Print and shaded views of the part. All mm, measured from the part's lowest x, y and z. A direction names the side the tool comes from. Coordinates: 2 decimals unless noted, no trailing zeros. Write each loop counter-clockwise with the first axis right and the second up, starting at its lowest first coordinate (ties: lowest second). Pieces come first, ordered by that corner, then holes. Notation, with made-up numbers: (-28.5, 38.5) -> (20.5, 38.5) arc R21 cw to (20.5, 61.5) -> close; hole circle Ø9 at (78, -27). An arc over 180 degrees is marked (long way). Write item = value, one per line.
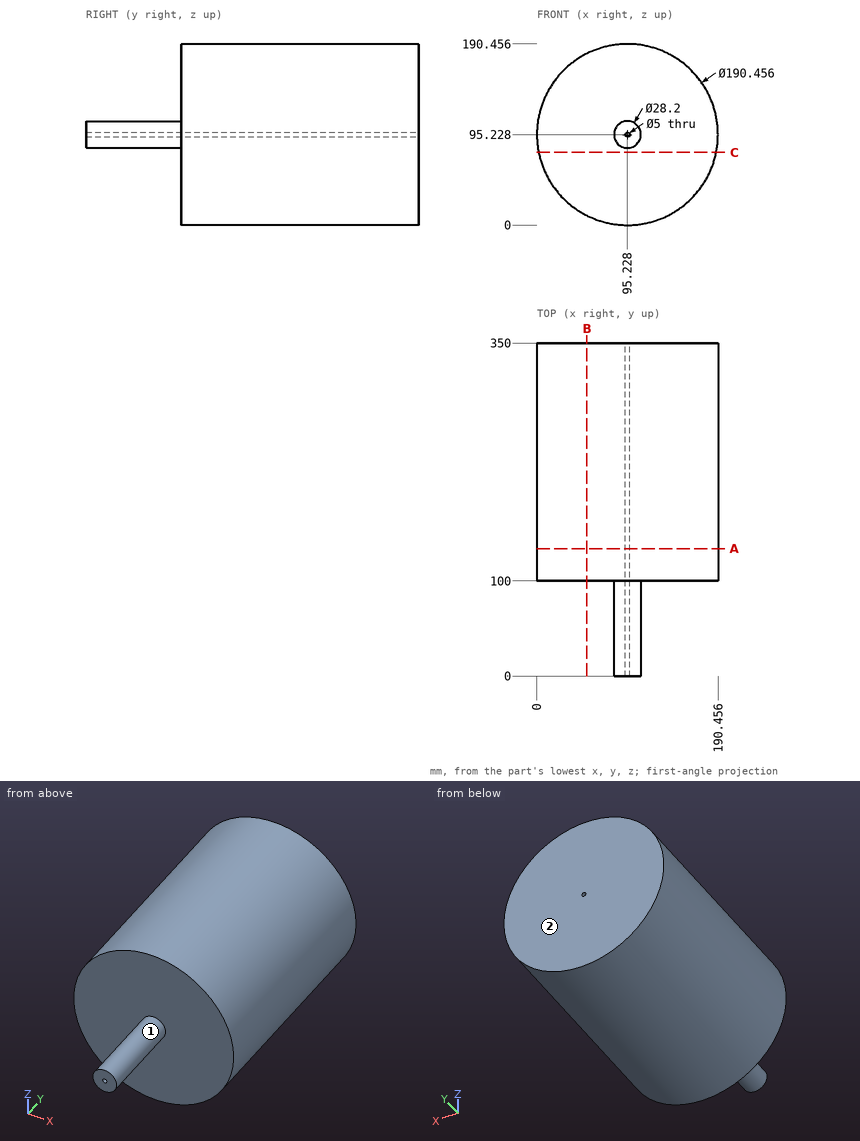
Q1. Saw through at C-C on z = 76.5. Give the cut face in (x, y) (1 decimal).
Model answer:
outline = (1.9, 100) -> (188.6, 100) -> (188.6, 350) -> (1.9, 350) -> close
Q2. Probe line 1 (Y direction, x = 72.5, z = 77); line 2 (X direction, y = 199, z = 54); line 3 (Z direction, x = 31, y = 292.5) (1 decimal). List the from-to ranges inside material, lowest first. Write a range as from..to.
Model answer:
line_1 = 100..350
line_2 = 9.39..181.07
line_3 = 24.9..165.5
Q3. Which spindle directions (+Z, -Z, +X, -X, +Y, -Y) get a long thin tool onto all of the face, cutting with end or side? Do the marked faces 1 and 2. Say none if no direction does.
Model answer:
face_1 = -Y
face_2 = +Z, -Z, +X, -X, +Y
Q4. Saw through at A-A on y = 134. Give the cut face in (x, z) (1 decimal).
Model answer:
outline = circle Ø190.5 at (95.2, 95.2); hole circle Ø5 at (95.2, 95.2)
Q5. Saw through at B-B on x = 52.5. Give the cut face in (y, z), and give its area (3 significant figures).
Model answer:
outline = (100, 10.12) -> (350, 10.12) -> (350, 180.33) -> (100, 180.33) -> close
area = 42,600 mm²
Q6. Pin check, flat tips, straight feed: pin 1 (10 mm diameter, centred on y = 206, z = 36.5, fed in from +X); pin 2 (2 mm diameter, centred on x = 55, z = 137.5, fed in from -Y); pin 3 (1 mm diameter, centred on x = 99.5, y = 271.5, fed in from +Z). Stop position of each tip, or through.
Model answer:
pin_1 = 173.85
pin_2 = 100
pin_3 = 190.38
